Geometry check sheet. Reference: the model listing, model coordinates, mm. Face numbers are marked on the shaded views. A direction names the side the tool comes from. Round coordinates to 2 decimals unless told otherwise and drop trailing zeros. Write each loop counter-clockwise with the first axis right and the second up, starting at its lowest first coordinate (ties: lowest second). Pieces come first, ordered by that corner, then holes. Notation, with made-up numbers: (56.25, -39) - (94.25, -39) arc R31 cw to (94.25, -5) - close; hole circle Ø8 at (46, 12). An arc over 180 degrees is marked (long way). One line per question, with ' | ' between items. Start each with the question number.
from build123d import *

# Parameters (mm, degrees)
SKETCH_1_W          = 60
SKETCH_1_H          = 150
EXTRUDE_1_DEPTH     = 30
SKETCH_2_R          = 5
CUT_EXTRUDE_1_DEPTH = 18
SKETCH_6_R          = 2
CUT_EXTRUDE_2_DEPTH = 83.758685345
EXTRUDE_2_DEPTH     = 60
SKETCH_8_W          = 60
SKETCH_8_H          = 30
EXTRUDE_3_DEPTH     = 60
SKETCH_9_W          = 139.095899212
SKETCH_9_H          = 109.690247042
CUT_EXTRUDE_3_DEPTH = 138.516765531
CUT_EXTRUDE_4_DEPTH = 221.495173564
EXTRUDE_4_DEPTH     = 30
CUT_EXTRUDE_5_DEPTH = 240.854663136


with BuildPart() as part:
    # 草图1 → 凸台-拉伸1 (new body)
    with BuildSketch(Plane.XY):
        Rectangle(SKETCH_1_W, SKETCH_1_H)
    extrude(amount=-EXTRUDE_1_DEPTH)

    # 草图2 → 切除-拉伸1 (cut)
    with BuildSketch(Plane(origin=(0, 0, -30), x_dir=(-1, 0, 0), z_dir=(0, 0, -1))):
        with Locations((-14.142135624, -35.857864376)):
            Circle(SKETCH_2_R)
        with Locations((14.142135624, -35.857864376)):
            Circle(SKETCH_2_R)
        with Locations((14.142135624, -64.142135624)):
            Circle(SKETCH_2_R)
        with Locations((-14.142135624, -64.142135624)):
            Circle(SKETCH_2_R)
    extrude(amount=-CUT_EXTRUDE_1_DEPTH, mode=Mode.SUBTRACT)

    # 草图6 → 切除-拉伸2 (cut, through all)
    with BuildSketch(Plane(origin=(0, 0, -12), x_dir=(-1, 0, 0), z_dir=(0, 0, -1))):
        with Locations((14.142135624, -64.142135624)):
            Circle(SKETCH_6_R)
        with Locations((-14.142135624, -64.142135624)):
            Circle(SKETCH_6_R)
        with Locations((-14.142135624, -35.857864376)):
            Circle(SKETCH_6_R)
        with Locations((14.142135624, -35.857864376)):
            Circle(SKETCH_6_R)
    extrude(amount=-CUT_EXTRUDE_2_DEPTH, mode=Mode.SUBTRACT)

    # 草图7 → 凸台-拉伸2 (add)
    with BuildSketch(Plane(origin=(30, 0, 0), x_dir=(0, 0, -1), z_dir=(1, 0, 0))):
        with BuildLine():
            Line((43.461758651, -132.675701756), (51.730879325, -103.837850878))
            ThreePointArc((51.730879325, -103.837850878), (36.040934699, -93.054450695), (30, -75))
            Line((30, -75), (0, -75))
            ThreePointArc((0, -75), (12.081869397, -111.108901389), (43.461758651, -132.675701756))
        make_face()
    extrude(amount=-EXTRUDE_2_DEPTH)

    # 草图8 → 凸台-拉伸3 (add)
    with BuildSketch(Plane(origin=(0, 0, -30), x_dir=(-1, 0, 0), z_dir=(0, 0, -1))):
        Rectangle(SKETCH_8_W, SKETCH_8_H)
    extrude(amount=EXTRUDE_3_DEPTH)

    # 草图9 → 切除-拉伸3 (cut, through all)
    with BuildSketch(Plane(origin=(0, -21.595774321, -75.313415293), x_dir=(-1, 0, 0), z_dir=(0, -0.27563735581699267, -0.9612616959383208))):
        Rectangle(SKETCH_9_W, SKETCH_9_H)
    extrude(amount=CUT_EXTRUDE_3_DEPTH, mode=Mode.SUBTRACT)

    # 草图10 → 切除-拉伸4 (cut, through all)
    with BuildSketch(Plane(origin=(30, -132.675701756, -43.461758651), x_dir=(-1, 0, 0), z_dir=(0, -0.9612616959383208, 0.27563735581699267))):
        with BuildLine():
            ThreePointArc((15.7, 0), (30, -14.3), (44.3, 0))
            Line((44.3, 0), (15.7, 0))
        make_face()
        with BuildLine():
            Line((15.7, 0), (44.3, 0))
            ThreePointArc((44.3, 0), (30, 14.3), (15.7, 0))
        make_face()
    extrude(amount=-CUT_EXTRUDE_4_DEPTH, mode=Mode.SUBTRACT)

    # 草图11 → 凸台-拉伸4 (add, symmetric)
    with BuildSketch(Plane(origin=(0, 0, 0), x_dir=(0, 0, -1), z_dir=(1, 0, 0))):
        with BuildLine():
            ThreePointArc((30, 75), (30.073078492, 77.092694212), (30.291957938, 79.175193029))
            Line((30.291957938, 79.175193029), (0.583915876, 83.350386058))
            ThreePointArc((0.583915876, 83.350386058), (0.146156984, 79.185388425), (0, 75))
            Line((0, 75), (30, 75))
        make_face()
    extrude(amount=EXTRUDE_4_DEPTH, both=True)

    # 草图12 → 切除-拉伸5 (cut, through all)
    with BuildSketch(Plane(origin=(30, 83.350386058, -0.583915876), x_dir=(1, 0, 0), z_dir=(0, 0.1391731009600656, 0.9902680687415703))):
        with BuildLine():
            ThreePointArc((-16, 0), (-30, 14), (-44, 0))
            Line((-44, 0), (-16, 0))
        make_face()
        with BuildLine():
            Line((-16, 0), (-44, 0))
            ThreePointArc((-44, 0), (-30, -14), (-16, 0))
        make_face()
    extrude(amount=-CUT_EXTRUDE_5_DEPTH, mode=Mode.SUBTRACT)


solid = part.part
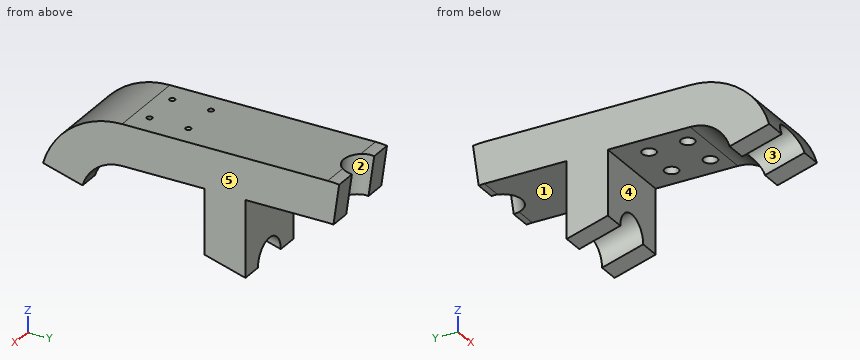
Q1. Section check C-C, the plane z = -58. Record the cut outline in (x, y), then the cut area to 3 significant figures.
Q2. Draft check along Y on the marked faces 1, 2 and 3. Enter one of: pulls with the +Y half, pulls with the -Y half, needs draft (parallel to the pull), parting line crosses it, or undercut.
Q3. Thickness scan on line 1 (Y direction, x = -18, z = -29.5); line 2 (X direction, y = -60, z = -18); line 3 (Z direction, x = -25.5, y = -56.5). Record the ranges inside material, lowest first.
Q4. Go/stop test with flat-tipped pins: P1, Ø12, axis at x = 10, z = -16, coming from the -Y side; P2, Ø3.5, axis at x = 14.14, y = -35.86, coming from the -Z side; P3, Ø11, axis at x = 13.5, y = -64, coming from the -Z side; P4, Ø5, axis at x = -13, y = -37, coming from the -Z side. Record where each tip stops, or that it passes through.
Q5. Section check A-A, the plane x = -22. Record the cut outline in (y, z), then the cut area to 3 significant figures.
Q6. Section check D-D, the plane z = -47.5. Count the separate pieces of the cut face and the enclosed holes in it, then the cut area to 3 significant figures.
Q7. Set-up check for the marked faces 4 and 5: record each of +Z, -Z, +X, -X, +Y, -Y from which the full face is reachable in a straight line by a thin tool's end or side.
Q8. Section check B-B, the plane y = 25.5. Record the cut outline in (x, z), then the cut area to 3 significant figures.
Result sheet:
1) outline: (-30, -15) - (30, -15) - (30, 15) - (-30, 15) - close | area: 1,800 mm²
2) face 1: undercut | face 2: pulls with the +Y half | face 3: pulls with the -Y half
3) line 1: -126.67 to -67.32, -60.96 to -39.04, -32.68 to 79.29 | line 2: -30 to -16.94, -11.34 to 11.34, 16.94 to 30 | line 3: -30 to 0
4) P1: y = -121.43 | P2: through | P3: z = -30 | P4: z = -12
5) outline: (-132.68, -43.46) - (-103.84, -51.73) arc R30 cw to (-75, -30) - (-15, -30) - (-15, -77.2) - (15, -85.81) - (15, -30) - (75, -30) arc R30 cw to (79.18, -30.29) - (83.35, -0.58) arc R60 ccw to (75, 0) - (-75, 0) arc R60 ccw to start | area: 7,980 mm²
6) separate pieces: 3 | enclosed holes: 0 | area: 2,320 mm²
7) face 4: -Z, +X, -X | face 5: +Z, -Z, +X, +Y, -Y
8) outline: (-30, -30) - (30, -30) - (30, 0) - (-30, 0) - close | area: 1,800 mm²
